Read the model definition and answer for the solid it produces. Units are mm, in the model's axes. A direction names the side the tool comes from. Give positions to 0.01 mm unless a question says otherwise; leave off trailing zeros. Write each loop counter-clockwise with the first axis right and the second up, starting at its lowest first coordinate (ties: lowest second). Pieces come first, ordered by that corner, then holes. Notation, with made-up numbers: (-11.75, 40.5) -> (15.25, 40.5) arc R26 cw to (15.25, 67.5) -> close; hole circle Ø8 at (80, 41.25). An arc over 180 degrees is marked (long way). Use a Markdown table: item, result.
Autodesk Inventor part; units mm, degrees
ref_plane "Płaszczyzna konstrukcyjna2" through (15, -111.85, 54) normal (0, 0, 1) x (1, 0, 0)
ref_plane "Płaszczyzna konstrukcyjna3" through (0, 0, 12) normal (0, 0, -1) x (-1, 0, 0)
ref_plane "YZ Plane" through (0, 0, 0) normal (1, 0, 0) x (0, 1, 0)
ref_plane "Płaszczyzna konstrukcyjna1" through (0, 0, 0) normal (0, 0, 1) x (1, 0, 0)
sketch "Szkic1" plane through (0, 0, 0) normal (0, 0, 1) x (1, 0, 0)
  arc A0 (15, -100.85) -> (100.85, -15) centre (0, 0) ccw
  arc A1 (15, -131.0443) -> (131.0443, -15) centre (0, 0) ccw
  line L0 (100.85, -15) -> (111.85, -15)
  line L1 (15, -100.85) -> (15, -111.85)
  line L2 (15.2, -100.8201) -> (15.2, -131.0213)
  line L3 (100.8201, -15.2) -> (131.0213, -15.2)
  point P0 (0, 0)
  dimension "d0" = 0.2
  dimension "d1" = 0.2
extrude "Wyciągnięcie proste1" add sketch "Szkic1" along normal up to surface (13.2464 mm away)
sketch "Szkic2" plane through (100.8201, -15.2, 13.2464) normal (0, 0, 1) x (1, 0, 0)
  line L0 (0, 0) -> (30.2012, 0)
  arc A0 (-85.6201, -85.6201) -> (0, 0) centre (-100.8201, 15.2) ccw
  line L1 (-85.6201, -115.8213) -> (-85.6201, -85.6201)
  arc A1 (-85.6201, -115.8213) -> (30.2012, 0) centre (-100.8201, 15.2) ccw
ref_plane "Płaszczyzna konstrukcyjna2" through (15, -111.85, 54) normal (0, 0, 1) x (1, 0, 0)
sketch "Szkic3" plane through (15, -111.85, 54) normal (0, 0, 1) x (1, 0, 0)
  arc A0 (0.2, 11.0299) -> (85.8201, 96.65) centre (-15, 111.85) ccw
  line L0 (0.2, -19.1713) -> (0.2, 11.0299)
  line L1 (85.8201, 96.65) -> (116.0213, 96.65)
  line L2 (0.2, 11.0299) -> (0.2, 0.0299)
  line L3 (0.2, -19.1713) -> (0.2, 11.0299)
  line L4 (85.8201, 96.65) -> (116.0213, 96.65)
  line L5 (85.8201, 96.65) -> (96.8201, 96.65)
  arc A1 (0.2, 0.0299) -> (96.8201, 96.65) centre (-49.8701, 146.7201) ccw
  point P0 (-15, 111.85)
  dimension "d4" = 11
  dimension "d5" = 11
  dimension "d6" = 155
loft "Wyciągnięcie złożone1" add profiles "Szkic2", "Szkic3"
sketch "Szkic7" plane through (0, 0, 0) normal (0, 0, -1) x (-1, 0, 0)
  line L0 (-109.9472, -18) -> (-109.9472, -15)
  line L1 (-108.4654, -20.2226) -> (-109.9472, -18)
  line L2 (-115.9472, -15) -> (-115.9472, -18)
  line L3 (-115.9472, -18) -> (-117.4289, -20.2226)
  arc A0 (-117.4289, -20.2226) -> (-117.0129, -21) centre (-117.0129, -20.5) ccw
  line L4 (-117.0129, -21) -> (-108.8814, -21)
  arc A1 (-108.8814, -21) -> (-108.4654, -20.2226) centre (-108.8814, -20.5) ccw
  line L5 (-100.8201, -15.2) -> (-131.0213, -15.2)
  line L6 (-18, -115.9472) -> (-15, -115.9472)
  line L7 (-20.2226, -117.4289) -> (-18, -115.9472)
  arc A2 (-21, -117.0129) -> (-20.2226, -117.4289) centre (-20.5, -117.0129) ccw
  line L8 (-21, -108.8814) -> (-21, -117.0129)
  arc A3 (-20.2226, -108.4654) -> (-21, -108.8814) centre (-20.5, -108.8814) ccw
  line L9 (-18, -109.9472) -> (-20.2226, -108.4654)
  line L10 (-15, -109.9472) -> (-18, -109.9472)
  line L11 (-15.2, -131.0213) -> (-15.2, -100.8201)
  line L12 (-15, -116.1472) -> (-17.9394, -116.1472)
  line L13 (-17.9394, -116.1472) -> (-20.1117, -117.5953)
  arc A4 (-21.2, -117.0129) -> (-20.1117, -117.5953) centre (-20.5, -117.0129) ccw
  line L14 (-21.2, -117.0129) -> (-21.2, -108.8814)
  arc A5 (-20.1117, -108.299) -> (-21.2, -108.8814) centre (-20.5, -108.8814) ccw
  line L15 (-20.1117, -108.299) -> (-17.9394, -109.7472)
  line L16 (-17.9394, -109.7472) -> (-15, -109.7472)
  line L17 (-109.7472, -15) -> (-109.7472, -17.9394)
  line L18 (-109.7472, -17.9394) -> (-108.299, -20.1117)
  arc A6 (-108.8814, -21.2) -> (-108.299, -20.1117) centre (-108.8814, -20.5) ccw
  line L19 (-108.8814, -21.2) -> (-117.0129, -21.2)
  arc A7 (-117.5953, -20.1117) -> (-117.0129, -21.2) centre (-117.0129, -20.5) ccw
  line L20 (-117.5953, -20.1117) -> (-116.1472, -17.9394)
  line L21 (-116.1472, -17.9394) -> (-116.1472, -15)
  line L22 (-116.1472, -15) -> (-109.7472, -15)
  line L23 (-15, -116.1472) -> (-15, -109.7472)
  point P0 (0, 0)
  dimension "d40" = 0.2
  dimension "d41" = 0.2
  dimension "d42" = 0.2
extrude "Wyciągnięcie proste6" cut sketch "Szkic7" against normal blind 31
sketch "Szkic5" plane through (0, 0, 0) normal (0, 0, -1) x (-1, 0, 0)
  circle A0 centre (-95.0216, -66.5349) radius 2.25
  circle A1 centre (-66.5349, -95.0216) radius 2.25
  point P0 (0, 0)
extrude "Wyciągnięcie proste4" cut sketch "Szkic5" against normal through all
ref_plane "Płaszczyzna konstrukcyjna3" through (0, 0, 12) normal (0, 0, -1) x (-1, 0, 0)
sketch "Szkic6" plane through (0, 0, 12) normal (0, 0, -1) x (-1, 0, 0)
  spline S0 degree 2 poles (-64.2849, -95.0216) (-64.2849, -91.1245) (-67.6599, -93.0731) (-71.0349, -95.0216) (-67.6599, -96.9702) (-64.2849, -98.9188) (-64.2849, -95.0216) knots 0 0 0 0.333333 0.333333 0.666667 0.666667 1 1 1 weights 1 0.5 1 0.5 1 0.5 1
  spline S1 degree 2 poles (-92.7716, -66.5349) (-92.7716, -62.6378) (-96.1466, -64.5863) (-99.5216, -66.5349) (-96.1466, -68.4834) (-92.7716, -70.432) (-92.7716, -66.5349) knots 0 0 0 0.333333 0.333333 0.666667 0.666667 1 1 1 weights 1 0.5 1 0.5 1 0.5 1
  circle A0 centre (-95.0216, -66.5349) radius 2.25
  circle A1 centre (-95.0216, -66.5349) radius 5
  circle A2 centre (-66.5349, -95.0216) radius 2.25
  circle A3 centre (-66.5349, -95.0216) radius 5
  point P0 (0, 0)
  dimension "d22" = 10
  dimension "d23" = 10
extrude "Wyciągnięcie proste5" cut sketch "Szkic6" against normal through all contours S0 | S1 | A1 | A3
equation "\"d1\" = d0"
properties part number "connectro_best"
Item 1: For a pull along Y with two mould halves and no side action, classify faces 1 (the face through (18, -113, 31)), 2 (the face through (94.138, -92.389, 6.53)), 3 (the face through (77, -77, 0)), 4 (the face through (109, -15.2, 27)) as +Y half, -Y half, draft (parallel to the pull), parting line (faces both ways), or undercut.
Return value:
| item | result |
|---|---|
| face 1 | undercut |
| face 2 | -Y half |
| face 3 | draft |
| face 4 | +Y half |
Item 2: Each of these flat-tipped pins is pushed along its axis until it touches: P1, Ø11, axis at x = 67, y = -94.5, coming from the +Z side; P2, Ø12, axis at y = -32.5, z = 26, coming from the +X side; P3, Ø4, axis at x = 95.02, y = -66.53, coming from the +Z side; P4, Ø3, axis at y = -39.5, z = 11, coming from the +X side. Where does it stop, or does it pass through?
Return value:
| item | result |
|---|---|
| P1 | z = 47.39 |
| P2 | x = 124.52 |
| P3 | through |
| P4 | x = 126.31 |
Item 3: A tool of negligible diameter and unlimited length cuts with its end or side. For faces 5 (the face through (17, -116.147, 15)), 6 (the face through (109.747, -17, 15)), 7 (the face through (113, -21.2, 15)), from which of +Z, -Z, +X, -X, +Y, -Y can it reach the whole face along a straight path? Write none if from no direction.
Return value:
| item | result |
|---|---|
| face 5 | -Z, -X |
| face 6 | -Z, +Y |
| face 7 | -Z |
Item 4: A cutting plane is placed at B-B (z = 29). Count the separate pieces of the cut face and the enclosed holes in it, then the cut area to 3 significant figures.
Return value:
| item | result |
|---|---|
| separate pieces | 1 |
| enclosed holes | 2 |
| area | 2,780 mm^2 |
Item 5: A cutting plane is placed at A-A (z = 4). Give the vertices of the cut face in (x, y).
Return value:
| item | result |
|---|---|
| outline | (15.2, -131.02) arc R131.9 ccw to (131.02, -15.2) -> (116.15, -15.2) -> (116.15, -17.94) -> (117.6, -20.11) arc R0.7 cw to (117.01, -21.2) -> (108.88, -21.2) arc R0.7 cw to (108.3, -20.11) -> (109.75, -17.94) -> (109.75, -15.2) -> (100.82, -15.2) arc R101.96 cw to (15.2, -100.82) -> (15.2, -109.75) -> (17.94, -109.75) -> (20.11, -108.3) arc R0.7 cw to (21.2, -108.88) -> (21.2, -117.01) arc R0.7 cw to (20.11, -117.6) -> (17.94, -116.15) -> (15.2, -116.15) -> close; hole circle Ø4.5 at (66.53, -95.02); hole circle Ø4.5 at (95.02, -66.53) |
Item 6: Straight lines are drawn through the part: line 1 along X through (y, z) = (-91.5, 29.5); line 2 along X through (y, z) = (-91.5, 23); line 3 along Y through (x, z) = (76, 50). For each, find the intervals that lie inside material, in ascending order. Write a range as [from, to].
Return value:
| item | result |
|---|---|
| line 1 | [44.98, 62.99], [70.08, 79.9] |
| line 2 | [44.98, 62.99], [70.08, 86.09] |
| line 3 | [-77.1, -67.97] |
